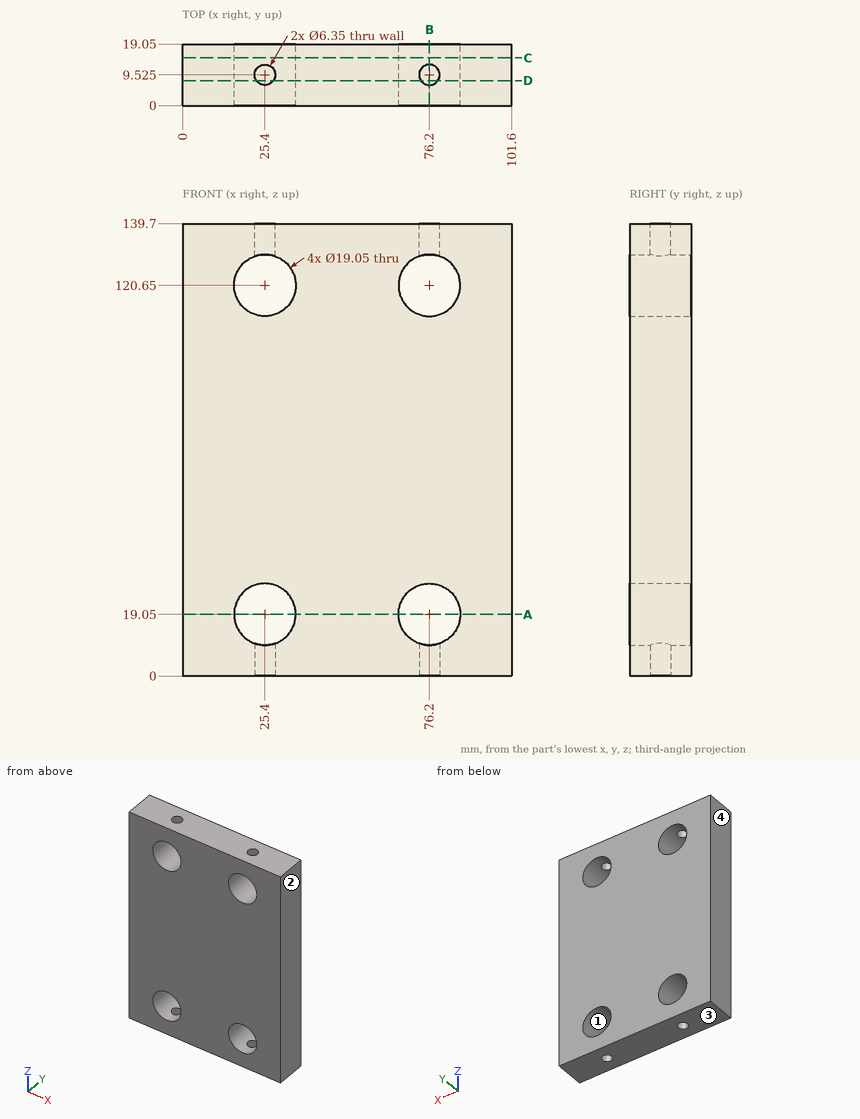
The drawing under review shows one solid part. Ordinate dimensions are in mm from its lowest x, y, z. Round coordinates to 2 decimals unless told otherwise and drop trailing zeros. Order: outer loops, then holes, each group sorted by start corner. A loop starts at its lowest first (then second) coordinate and runs counter-clockwise, first axis right, second up. Notation, with made-up numbers: M -34,-34 L -26,-34 A31 cw -26,-5 Z; hole C 57.5,80 d7. An arc over 180 degrees is marked long. Answer as CSV lines item,"result". Start each with the question number.
1) Add section D-D (y = 7.75). Give the boundary of the cut face in (x, z) (3 decimals).
2) Add section A-A (z = 19.05). Give the boundary of the cut face in (x, y) (3 decimals), then the cut area to 3 significant figures.
3) For pin 1 Ø11.5 at (x, z) = (76.2, 120.65) entering from -Y; pin 2 Ø5 at (x, y) = (76.2, 9.525) entering from +Z; pin 3 Ø4 at (x, y) = (25.4, 9.525) entering from -Z, all flat-tipped, find the tip position at first contact; note any pin that passes through.
4) Wall thickness on line 1 along X through (y, z) = (14, 19.05) (3 decimals); line 2 along Z through (x, y) = (72.5, 10.5); line 3 along X through (y, z) = (8.75, 6): over which ranges is each line inside the solid? List them lowest first. Write a range as [from, to].
5) The part is to be moulded in two halves that separate along X. For the marked faces 1, 2, 3 and 4, say which applies: +X half, -X half, draft (parallel to the pull), parting line (faces both ways), or undercut.
6) Add section B-B (x = 76.2). Give the boundary of the cut face in (y, z) (3 decimals), then the cut area to 3 significant figures.
7) Add section C-C (y = 14.75). Give the boundary of the cut face in (x, z) (3 decimals).
Resolved:
1,outline,"M 0,0 L 22.768,0 L 22.768,9.896 A9.525 cw long 28.032,9.896 L 28.032,0 L 73.568,0 L 73.568,9.896 A9.525 cw long 78.832,9.896 L 78.832,0 L 101.6,0 L 101.6,139.7 L 78.832,139.7 L 78.832,129.804 A9.525 cw long 73.568,129.804 L 73.568,139.7 L 28.032,139.7 L 28.032,129.804 A9.525 cw long 22.768,129.804 L 22.768,139.7 L 0,139.7 Z"
2,outline,"M 0,0 L 15.875,0 L 15.875,19.05 L 0,19.05 Z; M 34.925,0 L 66.675,0 L 66.675,19.05 L 34.925,19.05 Z; M 85.725,0 L 101.6,0 L 101.6,19.05 L 85.725,19.05 Z"
2,area,"1,210 mm^2"
3,pin 1,"through"
3,pin 2,"z = 111.46"
3,pin 3,"z = 28.36"
4,line 1,"[0, 15.875], [34.925, 66.675], [85.725, 101.6]"
4,line 2,"[0, 10.27], [27.83, 111.87], [129.43, 139.7]"
4,line 3,"[0, 22.32], [28.48, 73.12], [79.28, 101.6]"
5,face 1,"undercut"
5,face 2,"+X half"
5,face 3,"draft"
5,face 4,"-X half"
6,outline,"M 0,0 L 6.35,0 L 6.35,9.525 L 0,9.525 Z; M 0,28.575 L 19.05,28.575 L 19.05,111.125 L 0,111.125 Z; M 0,130.175 L 6.35,130.175 L 6.35,139.7 L 0,139.7 Z; M 12.7,0 L 19.05,0 L 19.05,9.525 L 12.7,9.525 Z; M 12.7,130.175 L 19.05,130.175 L 19.05,139.7 L 12.7,139.7 Z"
6,area,"1,810 mm^2"
7,outline,"M 0,0 L 101.6,0 L 101.6,139.7 L 0,139.7 Z; hole C 25.4,19.05 d19.05; hole C 25.4,120.65 d19.05; hole C 76.2,19.05 d19.05; hole C 76.2,120.65 d19.05"
